Geometry: final body of the model. Coordinates: model frame, mm. Round coordinates to 2 decimals unless told otherwise and drop trailing zeros. Loops run counter-clockwise (first coordinate to the right, second up) from the corner with the lowest first, then second, coordinate; pieces in that order, holes last. Notation, with made-up numbers: (-34.5, 18) -> (-30.5, 18) arc R35 ccw to (-30.5, 50) -> close; hole circle Ø9 at (44.5, 8.25). An arc over 180 degrees is marked (long way). Answer in a Markdown table with one row per item.
```python
from build123d import *

# Parameters (mm, degrees)
F1_DEPTH = 6.35
F2_D     = 3.4544


with BuildPart() as f1:
    # F0 (on Front) → F1 (new body)
    with BuildSketch(Plane.XZ):
        with BuildLine():
            ThreePointArc((4.9175919376, 4.0174356914), (2.012722134, 6.0225783192), (-1.5140395271, 6.1668617878))
            ThreePointArc((-1.5140395271, 6.1668617878), (-3.9184403149, -4.9968315459), (6.35, 0))
            ThreePointArc((6.35, 0), (6.3059786125, 0.746413919), (6.1745248068, 1.4824788061))
            ThreePointArc((6.1745248068, 1.4824788061), (4.4135292626, 2.1884040834), (4.9175919376, 4.0174356914))
        make_face()
    extrude(amount=F1_DEPTH)

    # F2 (through all)
    with Locations(Plane(origin=(0, 0, 0), x_dir=(1, 0, 0), z_dir=(0, 1, 0))):
        with Locations((0, 0)):
            Hole(F2_D / 2)


solid = f1.part
```
Item 1: First-contact query: P1, Ø1.5, axis at y = -5, z = 4.5, coming from the -X side. Flat tip, straight axial feed; report the tip coordinate or a pass-through.
Ans:
| item | result |
|---|---|
| P1 | x = -5.12 |
Item 2: Section query A-A, the plane x = 0. Output: boundary loops of the cut face in (y, z), and give its area (3 significant figures).
Ans:
| item | result |
|---|---|
| outline | (-6.35, -6.35) -> (0, -6.35) -> (0, -1.73) -> (-6.35, -1.73) -> close; (-6.35, 1.73) -> (0, 1.73) -> (0, 6.35) -> (-6.35, 6.35) -> close |
| area | 58.7 mm2 |
Item 3: Section query C-C, the plane z = -0.25. Output: boundary loops of the cut face in (x, y), and give its area (3 significant figures).
Ans:
| item | result |
|---|---|
| outline | (-6.35, -6.35) -> (-1.71, -6.35) -> (-1.71, 0) -> (-6.35, 0) -> close; (1.71, -6.35) -> (6.35, -6.35) -> (6.35, 0) -> (1.71, 0) -> close |
| area | 58.9 mm2 |
Item 4: Ray query, L1, parallel to Z at x = 0, y = -2.75; L2, parallel to X at y = -4, z = -1.25; L3, parallel to Z at x = 2, y = -3.75. Return the intervals inside material, ascending.
Ans:
| item | result |
|---|---|
| L1 | -6.35 to -1.73, 1.73 to 6.35 |
| L2 | -6.23 to -1.19, 1.19 to 6.23 |
| L3 | -6.03 to 6.03 |
Item 5: Mould query, pull axis X, two halves, no side actions, for faces 1 (the cylindrical face through (0.225, -3.219, -1.713)), 2 (the flat face through (-2, 0, -1)). Classes: released by +X, released by -X, zero draft, split by the parting line, or undercut.
Ans:
| item | result |
|---|---|
| face 1 | undercut |
| face 2 | zero draft |
Item 6: Section query B-B, the plane y = -2. Output: boundary loops of the cut face in (x, z).
Ans:
| item | result |
|---|---|
| outline | (4.92, 4.02) arc R6.35 ccw (long way) to (6.17, 1.48) arc R1.42 cw to start; hole circle Ø3.45 at (0, 0) |
Item 7: Section query D-D, the plane z = 2.5. Output: boundary loops of the cut face in (x, y).
Ans:
| item | result |
|---|---|
| outline | (-5.84, -6.35) -> (4.3, -6.35) -> (4.3, 0) -> (-5.84, 0) -> close |
